The model under review builds one solid part; all positions refer to its coordinate system, in mm. Face numbers are marked on the shaded views. A direction names the side the tool comes from. Give positions to 0.01 mm unless a question says otherwise; leave off trailing zeros. Order: outer loops, then holes, each group sorted by start corner. A loop starts at its lowest first (then second) coordinate and runs counter-clockwise, first axis right, second up. Notation, with made-up numbers: (17.25, 85.5) - (26.25, 85.5) arc R22 ccw to (26.25, 113.5) - close; hole circle Ø10 at (18, 15.25). An arc over 180 degrees is marked (long way). Put each result on its own line as item: value.
```python
from build123d import *

# Parameters (mm, degrees)
SALIENTE_EXTRUIR2_DEPTH = 10
CROQUIS9_W              = 24
CROQUIS9_H              = 7
CORTAR_EXTRUIR2_DEPTH   = 5
REDONDEO3_R             = 2.5


with BuildPart() as part:
    # Croquis1 → Saliente-Extruir2 (new body)
    with BuildSketch(Plane.XY):
        with BuildLine():
            ThreePointArc((-38.687161159, 0.254415054), (-39.39426794, 0.547308273), (-39.687161159, 1.254415054))
            Line((-39.687161159, 1.254415054), (-39.687161159, 24.254415054))
            ThreePointArc((-39.687161159, 24.254415054), (-39.39426794, 24.961521836), (-38.687161159, 25.254415054))
            Line((-38.687161159, 25.254415054), (-1.187161159, 25.254415054))
            Line((-1.187161159, 25.254415054), (-1.187161159, 28.254415054))
            Line((-1.187161159, 28.254415054), (-39.187161159, 28.254415054))
            ThreePointArc((-39.187161159, 28.254415054), (-42.015588284, 27.082842179), (-43.187161159, 24.254415054))
            Line((-43.187161159, 24.254415054), (-43.187161159, -3.245584946))
            Line((-43.187161159, -3.245584946), (-43.187161159, -4.245584946))
            ThreePointArc((-43.187161159, -4.245584946), (-44.358734034, -7.07401207), (-47.187161159, -8.245584946))
            Line((-47.187161159, -8.245584946), (-55.187161159, -8.245584946))
            Line((-55.187161159, -8.245584946), (-55.187161159, -11.745584946))
            Line((-55.187161159, -11.745584946), (-43.187161159, -11.745584946))
            Line((-43.187161159, -11.745584946), (-39.687161159, -11.745584946))
            Line((-39.687161159, -11.745584946), (-39.687161159, -5.245584946))
            ThreePointArc((-39.687161159, -5.245584946), (-39.101374721, -3.831371383), (-37.687161159, -3.245584946))
            Line((-37.687161159, -3.245584946), (-1.187161159, -3.245584946))
            Line((-1.187161159, -3.245584946), (-1.187161159, 0.254415054))
            Line((-1.187161159, 0.254415054), (-38.687161159, 0.254415054))
        make_face()
    saliente_extruir2 = extrude(amount=SALIENTE_EXTRUIR2_DEPTH)

    # Simetría2: Saliente-Extruir2 across plane
    add(saliente_extruir2.mirror(Plane(origin=(-1.187161159, 0, 10), x_dir=(0, 0, 1), z_dir=(-1, 0, 0))))

    # Croquis9 → Cortar-Extruir2 (cut)
    with BuildSketch(Plane.XY.offset(10)):
        with Locations((-1.187161159, -3.245584946)):
            Rectangle(CROQUIS9_W, CROQUIS9_H)
    extrude(amount=-CORTAR_EXTRUIR2_DEPTH, mode=Mode.SUBTRACT)

    # Redondeo3
    redondeo3_edges = [part.edges().sort_by_distance(p)[0] for p in [
        (10.812838841, -1.495584946, 5),
        (-13.187161159, -1.495584946, 5),
    ]]
    fillet(redondeo3_edges, radius=REDONDEO3_R)
    redondeo3_2_edges = [part.edges().sort_by_distance(p)[0] for p in [
        (10.812838841, -1.495584946, 10),
        (-13.187161159, -1.495584946, 10),
    ]]
    fillet(redondeo3_2_edges, radius=REDONDEO3_R - 0.0001)  # a hair under: the kernel refuses the full size


solid = part.part
```
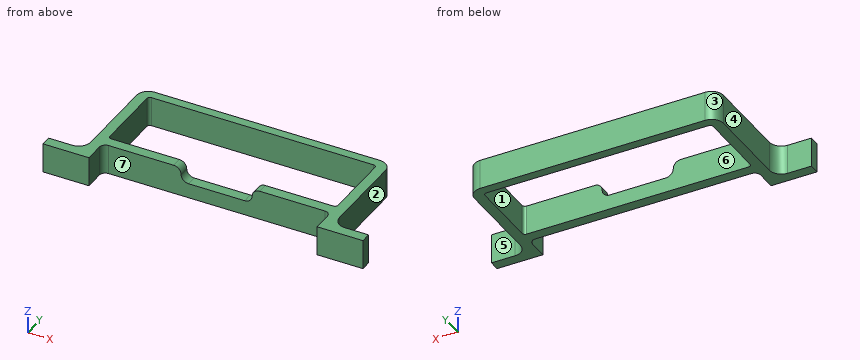
(1) Wall thickness on L1, parallel to Y at x = -33.5, z = 7; L2, parallel to X at y = 13.5, z = 0.5; L3, parallel to Y at x = 48, z = 9.75: over which ranges is each line inside the solid? List them lowest first.
The answers:
L1: -3.25 to 0.25, 25.25 to 28.25
L2: -43.19 to -39.69, 37.31 to 40.81
L3: -11.75 to -8.25
(2) Take a section at C-C, the plane x = -22. Write out the cut boundary in (y, z), then the cut area to 3 significant figures.
The answers:
outline: (-3.25, 0) - (0.25, 0) - (0.25, 10) - (-3.25, 10) - close; (25.25, 0) - (28.25, 0) - (28.25, 10) - (25.25, 10) - close
area: 65.0 mm^2
(3) Take a section at B-B, the plane z = 2. Write out the cut boundary in (x, y), then the cut area to 3 significant figures.
The answers:
outline: (-55.19, -11.75) - (-39.69, -11.75) - (-39.69, -5.25) arc R2 cw to (-37.69, -3.25) - (35.31, -3.25) arc R2 cw to (37.31, -5.25) - (37.31, -11.75) - (52.81, -11.75) - (52.81, -8.25) - (44.81, -8.25) arc R4 cw to (40.81, -4.25) - (40.81, 24.25) arc R4 ccw to (36.81, 28.25) - (-39.19, 28.25) arc R4 ccw to (-43.19, 24.25) - (-43.19, -4.25) arc R4 cw to (-47.19, -8.25) - (-55.19, -8.25) - close; hole (-39.69, 1.25) arc R1 ccw to (-38.69, 0.25) - (36.31, 0.25) arc R1 ccw to (37.31, 1.25) - (37.31, 24.25) arc R1 ccw to (36.31, 25.25) - (-38.69, 25.25) arc R1 ccw to (-39.69, 24.25) - close
area: 867 mm^2
(4) Clearance check with flat-ended pins moving along their axes: pin 1 Ø3 at (y, z) = (3, 5.5) entering from -X; pin 2 Ø3 at (y, z) = (9.5, 3.5) entering from +X; pin 3 Ø3 at (x, z) = (10, 4) entering from -Y. State where each tip first meets the part, or that it passes through.
The answers:
pin 1: x = -43.19
pin 2: x = 40.81
pin 3: y = -3.25
(5) For the marked faces 4, 5, 6 and 7, list the 3-axis set-ups (+Z, -Z, +X, -X, +Y, -Y) from which the entire face can be reached by the end or side of a thin tool; tool diameter is ignored.
The answers:
face 4: +Z, -Z, -X, +Y
face 5: +Z, -Z, +X, +Y
face 6: +Z, -Z
face 7: +Z, -Z, -Y
(6) Take a section at A-A, the plane y = 10. Write out the cut boundary in (x, z), then the cut area to 3 significant figures.
The answers:
outline: (-43.19, 0) - (-39.69, 0) - (-39.69, 10) - (-43.19, 10) - close; (37.31, 0) - (40.81, 0) - (40.81, 10) - (37.31, 10) - close
area: 70.0 mm^2
(7) The part is to be moulded in two halves that separate along Y. For the marked faces 1, 2 and 3, say which applies: pulls with the +Y half, pulls with the -Y half, needs draft (parallel to the pull), parting line crosses it, or undercut.
The answers:
face 1: undercut
face 2: needs draft
face 3: pulls with the +Y half
